from build123d import *

# Parameters (mm, degrees)
F0_R      = 8.5
F1_DEPTH  = 4
F3_R      = 5
F4_DEPTH  = 100
F5_W      = 4
F5_H      = 5
F9_DEPTH  = 3
F10_R     = 1.5
F11_DEPTH = 118.9


with BuildPart() as f1:
    # F0 (on Top) → F1 (new body)
    with BuildSketch(Plane.XY):
        Circle(F0_R)
    extrude(amount=F1_DEPTH)

    # F3 (on Top) → F4 (join)
    with BuildSketch(Plane.XY):
        Circle(F3_R)
    extrude(amount=F4_DEPTH)

    # F5 (on Right) → F6 (revolve)
    with BuildSketch(Plane.YZ):
        with Locations((2, 102.5)):
            Rectangle(F5_W, F5_H)
    revolve(axis=Axis((0, 0, 102.5), (0, 0, -1)))

    # F8 (on face) → F9 (cut)
    with BuildSketch(Plane.XY.offset(105)):
        with BuildLine():
            Line((3.8729833462, 1), (1, 1))
            Line((1, 1), (1, -1))
            Line((1, -1), (3.8729833462, -1))
            ThreePointArc((3.8729833462, -1), (3.9681187851, -0.5040171699), (4, 0))
            ThreePointArc((4, 0), (3.9681187851, 0.5040171699), (3.8729833462, 1))
        make_face()
    extrude(amount=-F9_DEPTH, mode=Mode.SUBTRACT)

    # F10 (on face) → F11 (cut)
    with BuildSketch(Plane.XY.offset(105)):
        Circle(F10_R)
    extrude(amount=-F11_DEPTH, mode=Mode.SUBTRACT)


solid = f1.part
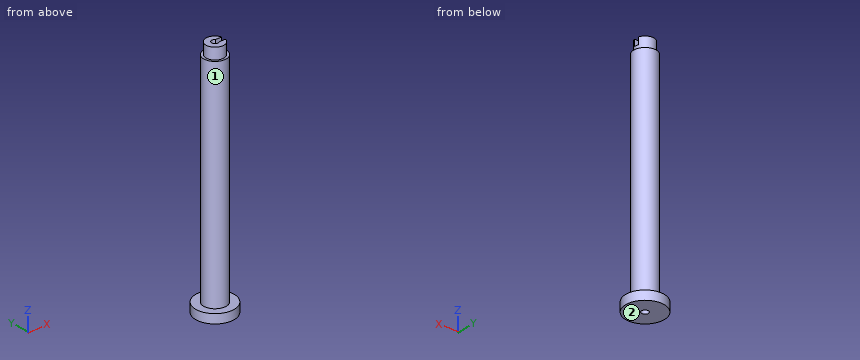
Geometry check sheet. Reference: the model listing, model coordinates, mm. Face numbers are marked on the shaded views. A direction names the side the tool comes from. Give positions to 0.01 mm unless a question says otherwise; leave off trailing zeros. Write each loop counter-clockwise with the first axis right and the second up, starting at its lowest first coordinate (ties: lowest second). Pieces come first, ordered by that corner, then holes.
1) Set-up check for the marked faces 1 and 2: record each of +Z, -Z, +X, -X, +Y, -Y from which the full face is reachable in a straight line by a thin tool's end or side.
Values follow:
face 1: +Z
face 2: -Z, +X, -X, +Y, -Y
2) Cross-section at B-B (x = 0). Record the boundary of the cut face in (y, z), plus the area to 3 significant figures.
Values follow:
outline: (-8.5, 0) - (-1.5, 0) - (-1.5, 105) - (-4, 105) - (-4, 100) - (-5, 100) - (-5, 4) - (-8.5, 4) - close; (1.5, 0) - (8.5, 0) - (8.5, 4) - (5, 4) - (5, 100) - (4, 100) - (4, 105) - (1.5, 105) - close
area: 753 mm2
3) Thickness scan on line 1 (Y direction, x = 0, z = 82.5); line 2 (Z direction, x = 6.5, y = -2.75). Record the ranges inside material, lowest first.
Values follow:
line 1: y = -5 to -1.5, 1.5 to 5
line 2: z = 0 to 4
4) Cross-section at D-D (x = -7). Record the boundary of the cut face in (y, z), plus the area to 3 significant figures.
Values follow:
outline: (-4.82, 0) - (4.82, 0) - (4.82, 4) - (-4.82, 4) - close
area: 38.6 mm2
5) Go/stop test with flat-tipped pins: pin 1 Ø0.6 at (x, y) = (2.5, 0) entering from +Z; pin 2 Ø1 at (y, z) = (0, 73) entering from -X; pin 3 Ø5 at (x, z) = (-6, 88) entering from -Y; pin 4 Ø1.8 at (x, y) = (0, 0) entering from +Z. Record where each tip stops, or that it passes through.
Values follow:
pin 1: stops at z = 102
pin 2: stops at x = -5
pin 3: stops at y = -3.57
pin 4: passes through
6) Cross-section at A-A (y = 0). Record the boundary of the cut face in (x, z), plus the area to 4 significant figures.
Values follow:
outline: (-8.5, 0) - (-1.5, 0) - (-1.5, 105) - (-4, 105) - (-4, 100) - (-5, 100) - (-5, 4) - (-8.5, 4) - close; (1.5, 0) - (8.5, 0) - (8.5, 4) - (5, 4) - (5, 100) - (4, 100) - (4, 102) - (1.5, 102) - close
area: 745.5 mm2
7) Cross-section at C-C (z = 64). Record the boundary of the cut face in (x, y), plus the area to 3 significant figures.
Values follow:
outline: circle Ø10 at (0, 0); hole circle Ø3 at (0, 0)
area: 71.5 mm2
